Geometry: final body of the model. Coordinates: model frame, mm. Face numbers are marked on the shaded views. A direction names the side the tool comes from. Round coordinates to 2 decimals unless told otherwise and drop trailing zeros. Write each loop counter-clockwise with the first axis right and the second up, starting at its lowest first coordinate (ties: lowest second). Pieces come first, ordered by that corner, then holes. Notation, with made-up numbers: (7, 5) - (47, 5) arc R21 cw to (47, 16) - close; hole circle Ø11 at (68.25, -30.5). An arc over 180 degrees is marked (long way). Write each question's results on one line, items separated by ' | '.
from build123d import *

# Parameters (mm, degrees)
F1_DEPTH = 25
F3_D     = 7.5
F4_D     = 7.5


with BuildPart() as f1:
    # F0 (on Front) → F1 (new body)
    with BuildSketch(Plane.XZ):
        with BuildLine():
            Line((-49.944923, 46.371131), (-54.944923, 46.371131))
            Line((-54.944923, 46.371131), (-54.944923, 41.371131))
            ThreePointArc((-54.944923, 41.371131), (-53.480457, 37.835597), (-49.944923, 36.371131))
            Line((-49.944923, 36.371131), (-32.461094, 36.371131))
            ThreePointArc((-32.461094, 36.371131), (-29.781383, 35.592405), (-27.936377, 33.498791))
            ThreePointArc((-27.936377, 33.498791), (-11.194923, 22.871131), (5.54653, 33.498791))
            ThreePointArc((5.54653, 33.498791), (7.391536, 35.592405), (10.071247, 36.371131))
            Line((10.071247, 36.371131), (27.555077, 36.371131))
            ThreePointArc((27.555077, 36.371131), (31.09061, 37.835597), (32.555077, 41.371131))
            Line((32.555077, 41.371131), (32.555077, 48.871131))
            Line((32.555077, 48.871131), (27.555077, 48.871131))
            Line((27.555077, 48.871131), (27.555077, 41.371131))
            Line((27.555077, 41.371131), (2.305077, 41.371131))
            ThreePointArc((2.305077, 41.371131), (-11.194923, 27.871131), (-24.694923, 41.371131))
            Line((-24.694923, 41.371131), (-49.944923, 41.371131))
            Line((-49.944923, 41.371131), (-49.944923, 46.371131))
        make_face()
    extrude(amount=F1_DEPTH)

    # F3 (through all)
    with Locations(Plane(origin=(0, 0, 36.371131), x_dir=(1, 0, 0), z_dir=(0, 0, -1))):
        with Locations((-41.203009, 12.5)):
            Hole(F3_D / 2)

    # F4 (through all)
    with Locations(Plane(origin=(0, 0, 36.371131), x_dir=(1, 0, 0), z_dir=(0, 0, -1))):
        with Locations((18.813162, 12.5)):
            Hole(F4_D / 2)


solid = f1.part
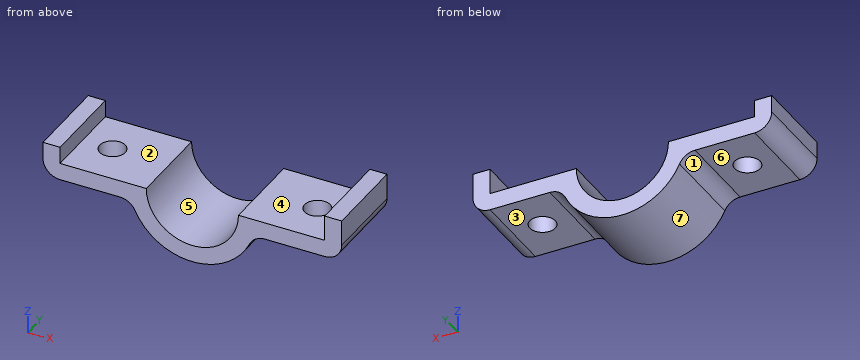
Q1. Access query for the marked faces 1, 2 and 3. Directions: +Z, -Z, +X, -X, +Y, -Y. A direction counts if a zero-diameter tool reaches every point of the face in a straight line with its end or side. Return the directions, or none.
Answer block:
face 1: -Z, -X, +Y, -Y | face 2: +Z, +Y, -Y | face 3: -Z, +X, +Y, -Y
Q2. Ray query, line 1 along X through (y, z) = (-19.25, 42); line 2 along X through (y, z) = (-18.25, 41); line 3 along X through (y, z) = (-2, 47.75). Return the intervals inside material, ascending.
Answer block:
line 1: -54.94 to -49.94, 27.56 to 32.56 | line 2: -54.93 to -24.69, 2.3 to 32.54 | line 3: 27.56 to 32.56
Q3. Mould query, pull axis X, two halves, no side actions, for the marked faces 4, 5, 6 and 7. Classes: pulls with the +X half, pulls with the -X half, needs draft (parallel to the pull), parting line crosses it, or undercut.
Answer block:
face 4: undercut | face 5: undercut | face 6: needs draft | face 7: parting line crosses it
Q4. Section query A-A, the plane z = 39. Return loops of the section in (x, y), plus the area to 3 significant figures.
Answer block:
outline: (-54.35, -25) - (-24.49, -25) - (-24.49, 0) - (-54.35, 0) - close; (2.1, -25) - (31.96, -25) - (31.96, 0) - (2.1, 0) - close; hole circle Ø7.5 at (-41.2, -12.5); hole circle Ø7.5 at (18.81, -12.5) | area: 1,400 mm2
Q5. Section query D-D, the plane y = -7.5. Return loops of the section in (x, z).
Answer block:
outline: (-54.94, 41.37) arc R5 ccw to (-49.94, 36.37) - (-32.46, 36.37) arc R5 cw to (-27.94, 33.5) arc R18.5 ccw to (5.55, 33.5) arc R5 cw to (10.07, 36.37) - (27.56, 36.37) arc R5 ccw to (32.56, 41.37) - (32.56, 48.87) - (27.56, 48.87) - (27.56, 41.37) - (2.31, 41.37) arc R13.5 cw to (-24.69, 41.37) - (-49.94, 41.37) - (-49.94, 46.37) - (-54.94, 46.37) - close
Q6. Section query B-B, the plane z = 42.5. Return loops of the section in (x, y), plus the area to 3 significant figures.
Answer block:
outline: (-54.94, -25) - (-49.94, -25) - (-49.94, 0) - (-54.94, 0) - close; (27.56, -25) - (32.56, -25) - (32.56, 0) - (27.56, 0) - close | area: 250 mm2
Q7. Section query C-C, the plane y = -12.5. Return loops of the section in (x, z), plus the area to 3 significant figures.
Answer block:
outline: (-54.94, 41.37) arc R5 ccw to (-49.94, 36.37) - (-44.95, 36.37) - (-44.95, 41.37) - (-49.94, 41.37) - (-49.94, 46.37) - (-54.94, 46.37) - close; (-37.45, 36.37) - (-32.46, 36.37) arc R5 cw to (-27.94, 33.5) arc R18.5 ccw to (5.55, 33.5) arc R5 cw to (10.07, 36.37) - (15.06, 36.37) - (15.06, 41.37) - (2.31, 41.37) arc R13.5 cw to (-24.69, 41.37) - (-37.45, 41.37) - close; (22.56, 36.37) - (27.56, 36.37) arc R5 ccw to (32.56, 41.37) - (32.56, 48.87) - (27.56, 48.87) - (27.56, 41.37) - (22.56, 41.37) - close | area: 487 mm2
Q8. Pin query (flat end, axial travel): pin 1 (10 mm diameter, centred on x = 11.5, z = 43, fed in from -Y); pin 2 (7.5 mm diameter, centred on x = -41.5, y = -8, fed in from +Z); pin 3 (6 mm diameter, centred on y = -11, z = 32, fed in from -X); pin 4 (12 mm diameter, centred on x = -41.2, y = -12.5, fed in from -Z). Return the tip coordinate at first contact, or that it passes through.
Answer block:
pin 1: y = -25 | pin 2: z = 41.37 | pin 3: x = -29.02 | pin 4: z = 36.37
